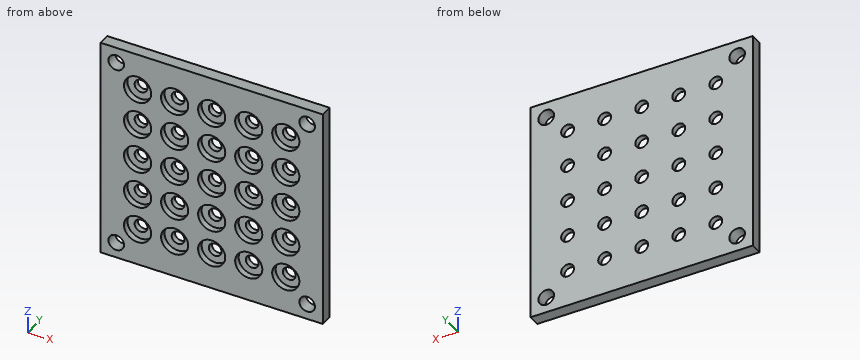
```python
from build123d import *

# Parameters (mm, degrees)
F0_W     = 90
F0_H     = 90
F0_R     = 3.175
F1_DEPTH = 4.77
F2_R     = 2.6
F3_DEPTH = 4.77
F4_R     = 5.5
F5_DEPTH = 2.5


with BuildPart() as f1:
    # F0 (on Front) → F1 (new body)
    with BuildSketch(Plane.XZ):
        Rectangle(F0_W, F0_H)
        with Locations((-38.65, -38.65)):
            Circle(F0_R, mode=Mode.SUBTRACT)
        with Locations((38.65, -38.65)):
            Circle(F0_R, mode=Mode.SUBTRACT)
        with Locations((-38.65, 38.65)):
            Circle(F0_R, mode=Mode.SUBTRACT)
        with Locations((38.65, 38.65)):
            Circle(F0_R, mode=Mode.SUBTRACT)
    extrude(amount=F1_DEPTH)

    # F2 (on face) → F3 (cut, through all)
    with BuildSketch(Plane.XZ.offset(4.77)):
        with Locations((-30, 30)):
            Circle(F2_R)
        with Locations((-30, 15)):
            Circle(F2_R)
        with Locations((-30, 0)):
            Circle(F2_R)
        with Locations((-30, -15)):
            Circle(F2_R)
        with Locations((-30, -30)):
            Circle(F2_R)
        with Locations((-15, 30)):
            Circle(F2_R)
        with Locations((-15, 15)):
            Circle(F2_R)
        with Locations((-15, 0)):
            Circle(F2_R)
        with Locations((-15, -15)):
            Circle(F2_R)
        with Locations((-15, -30)):
            Circle(F2_R)
        with Locations((0, 30)):
            Circle(F2_R)
        with Locations((0, 15)):
            Circle(F2_R)
        Circle(F2_R)
        with Locations((0, -15)):
            Circle(F2_R)
        with Locations((0, -30)):
            Circle(F2_R)
        with Locations((15, 30)):
            Circle(F2_R)
        with Locations((15, 15)):
            Circle(F2_R)
        with Locations((15, 0)):
            Circle(F2_R)
        with Locations((15, -15)):
            Circle(F2_R)
        with Locations((15, -30)):
            Circle(F2_R)
        with Locations((30, 30)):
            Circle(F2_R)
        with Locations((30, 15)):
            Circle(F2_R)
        with Locations((30, 0)):
            Circle(F2_R)
        with Locations((30, -15)):
            Circle(F2_R)
        with Locations((30, -30)):
            Circle(F2_R)
    extrude(amount=-F3_DEPTH, mode=Mode.SUBTRACT)

    # F4 (on face) → F5 (cut)
    with BuildSketch(Plane.XZ.offset(4.77)):
        with Locations((-30, 30)):
            Circle(F4_R)
        with Locations((-30, 15)):
            Circle(F4_R)
        with Locations((-30, 0)):
            Circle(F4_R)
        with Locations((-30, -15)):
            Circle(F4_R)
        with Locations((-30, -30)):
            Circle(F4_R)
        with Locations((-15, 30)):
            Circle(F4_R)
        with Locations((-15, 15)):
            Circle(F4_R)
        with Locations((-15, 0)):
            Circle(F4_R)
        with Locations((-15, -15)):
            Circle(F4_R)
        with Locations((-15, -30)):
            Circle(F4_R)
        with Locations((0, 30)):
            Circle(F4_R)
        with Locations((0, 15)):
            Circle(F4_R)
        Circle(F4_R)
        with Locations((0, -15)):
            Circle(F4_R)
        with Locations((0, -30)):
            Circle(F4_R)
        with Locations((15, 30)):
            Circle(F4_R)
        with Locations((15, 15)):
            Circle(F4_R)
        with Locations((15, 0)):
            Circle(F4_R)
        with Locations((15, -15)):
            Circle(F4_R)
        with Locations((15, -30)):
            Circle(F4_R)
        with Locations((30, 30)):
            Circle(F4_R)
        with Locations((30, 15)):
            Circle(F4_R)
        with Locations((30, 0)):
            Circle(F4_R)
        with Locations((30, -15)):
            Circle(F4_R)
        with Locations((30, -30)):
            Circle(F4_R)
    extrude(amount=-F5_DEPTH, mode=Mode.SUBTRACT)


solid = f1.part
```
Can you work these out from the model? Positions are in its coordinate system, mm. Give positions to 0.01 mm unless a question says otherwise; leave off trailing zeros. Order: outer loops, then holes, each group sorted by start corner. A loop starts at its lowest first (then second) coordinate and runs counter-clockwise, first axis right, second up. Notation, with made-up numbers: M -31.5,13.25 L -9.5,13.25 A27 ccw -9.5,35.25 Z; hole C -39.75,14.25 d7. An arc over 180 degrees is marked long. One line per item, written item: value.
1) Please list where these lines run through material, in increasing order: line 1 along Z through (x, y) = (15, -1.05); line 2 along Z through (x, y) = (15, -4.1); line 3 along X through (y, z) = (-1.6, -14).
Answer sheet:
line 1: z = -45 to -32.6, -27.4 to -17.6, -12.4 to -2.6, 2.6 to 12.4, 17.6 to 27.4, 32.6 to 45
line 2: z = -45 to -35.5, -24.5 to -20.5, -9.5 to -5.5, 5.5 to 9.5, 20.5 to 24.5, 35.5 to 45
line 3: x = -45 to -32.4, -27.6 to -17.4, -12.6 to -2.4, 2.4 to 12.6, 17.4 to 27.6, 32.4 to 45
2) I want a section at B-B, the plane y = -3.85. Count the separate pieces of the cut face and the enclosed holes in it, plus the area to 3 significant figures.
Answer sheet:
separate pieces: 1
enclosed holes: 29
area: 5,600 mm^2
3) I want a section at A-A, the plane z = -38.65. List the corners of the cut face in (x, y) for me (3 decimals), plus the area to 3 significant figures.
Answer sheet:
outline: M -45,-4.77 L -41.825,-4.77 L -41.825,0 L -45,0 Z; M -35.475,-4.77 L 35.475,-4.77 L 35.475,0 L -35.475,0 Z; M 41.825,-4.77 L 45,-4.77 L 45,0 L 41.825,0 Z
area: 369 mm^2
4) For P1, Ø6.5, axis at x = 15, z = -15, coming from the -Y side, with a flat end and sliding along its axis, tell me the tip position at first contact or that it passes through.
Answer sheet:
P1: stops at y = -2.27
